The listing builds one solid part. Answer for the finished solid, in the listing's coordinates (mm). Face numbers are marked on the shaded views. A direction names the side the tool comes from. Coordinates: 2 decimals unless noted, no trailing zeros. Order: outer loops, then holes, each group sorted by start corner. A loop starts at its lowest first (then second) coordinate and runs counter-clockwise, first axis right, second up. Notation, with made-up numbers: (19, 9.25) -> (78, 9.25) arc R23 cw to (78, 33.25) -> close; hole circle Ø6 at (-40, 3.25). An arc over 180 degrees is marked (long way). One line per question, with ' | ' between items.
from build123d import *

# Parameters (mm, degrees)
F0_W     = 110.95576
F0_H     = 66.701726
F1_DEPTH = 62.738
F2_R     = 5.600926
F3_DEPTH = 110.95676
F4_W     = 99.779762
F4_H     = 55.525728
F5_DEPTH = 62.739
F6_W     = 47.409441
F6_H     = 21.149314
F7_DEPTH = 66.702725


with BuildPart() as f1:
    # F0 (on Top) → F1 (new body)
    with BuildSketch(Plane.XY):
        Rectangle(F0_W, F0_H)
    extrude(amount=F1_DEPTH)

    # F2 (on face) → F3 (cut, through all)
    with BuildSketch(Plane.YZ.offset(55.47788)):
        with Locations((0, 31.369)):
            Circle(F2_R)
    extrude(amount=-F3_DEPTH, mode=Mode.SUBTRACT)

    # F4 (on face) → F5 (cut, through all)
    with BuildSketch(Plane.XY.offset(62.738)):
        Rectangle(F4_W, F4_H)
    extrude(amount=-F5_DEPTH, mode=Mode.SUBTRACT)

    # F6 (on face) → F7 (cut, through all)
    with BuildSketch(Plane.XZ.offset(33.350863)):
        with Locations((0.224762, 52.163343)):
            Rectangle(F6_W, F6_H)
    extrude(amount=-F7_DEPTH, mode=Mode.SUBTRACT)


solid = f1.part
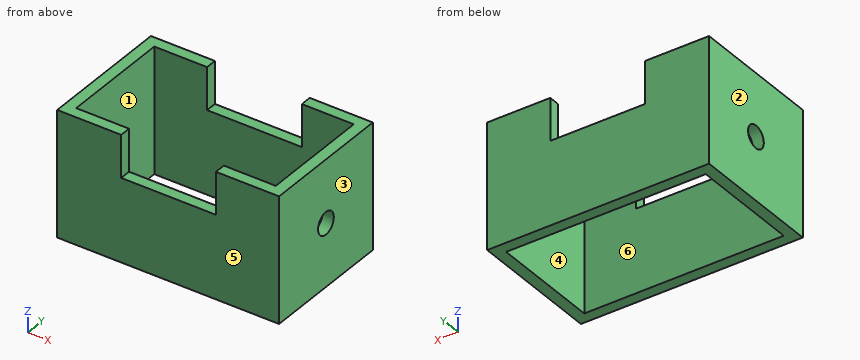
Item 1: Section C-C, the plane z = 8.5 is taken. Give the vertices of the cut face in (x, y), plus the area to 3 significant figures.
Computed values:
outline: (-55.48, -33.35) -> (55.48, -33.35) -> (55.48, 33.35) -> (-55.48, 33.35) -> close; hole (-49.89, -27.76) -> (49.89, -27.76) -> (49.89, 27.76) -> (-49.89, 27.76) -> close | area: 1,860 mm^2
Item 2: For the marked faces 1 and 2, determine the directions among +Z, -Z, +X, -X, +Y, -Y from which every point of the face is accessible in a straight line to the end or side of a thin tool.
Computed values:
face 1: +Z, -Z | face 2: +Z, -Z, -X, +Y, -Y
Item 3: This flat-tipped pin is pushed along its axis until it touches: pin 1 Ø1.7 at (x, y) = (0.5, -30.5) entering from +Z. Where does it stop, or does it pass through?
Computed values:
pin 1: stops at z = 41.59
Item 4: Find the intervals of material crossed by L1, parallel to Y at x = 14, z = 28; L2, parallel to Z at x = -54.3, y = 0; L3, parallel to X at y = 6, z = 51, in increasing order.
Computed values:
L1: y = -33.35 to -27.76, 27.76 to 33.35 | L2: z = 0 to 25.77, 36.97 to 62.74 | L3: x = -55.48 to -49.89, 49.89 to 55.48
Item 5: Section D-D, the plane y = -14 is taken. Give the vertices of the cut face in (x, z).
Computed values:
outline: (-55.48, 0) -> (-49.89, 0) -> (-49.89, 62.74) -> (-55.48, 62.74) -> close; (49.89, 0) -> (55.48, 0) -> (55.48, 62.74) -> (49.89, 62.74) -> close
Item 6: Section A-A, the plane x = 28 is taken. Give the vertices of the cut face in (y, z).
Computed values:
outline: (-33.35, 0) -> (-27.76, 0) -> (-27.76, 62.74) -> (-33.35, 62.74) -> close; (27.76, 0) -> (33.35, 0) -> (33.35, 62.74) -> (27.76, 62.74) -> close
Item 7: Section B-B, the plane y = 0 is taken. Give the vertices of the cut face in (x, z), plus the area to 3 significant figures.
Computed values:
outline: (-55.48, 0) -> (-49.89, 0) -> (-49.89, 25.77) -> (-55.48, 25.77) -> close; (-55.48, 36.97) -> (-49.89, 36.97) -> (-49.89, 62.74) -> (-55.48, 62.74) -> close; (49.89, 0) -> (55.48, 0) -> (55.48, 25.77) -> (49.89, 25.77) -> close; (49.89, 36.97) -> (55.48, 36.97) -> (55.48, 62.74) -> (49.89, 62.74) -> close | area: 576 mm^2
Item 8: Determine the mould class of the marked faces 3, 4, 5 and 6 for opening direction X: pulls with the +X half, pulls with the -X half, needs draft (parallel to the pull), parting line crosses it, or undercut.
Computed values:
face 3: pulls with the +X half | face 4: undercut | face 5: needs draft | face 6: undercut
